```python
from build123d import *

# Parameters (mm, degrees)
F0_R      = 15.875
F0_R_2    = 12.7
F1_DEPTH  = 6.35
F2_W      = 31.75
F2_H      = 25.4
F3_DEPTH  = 6.35
F4_W      = 31.75
F4_H      = 6.35
F5_DEPTH  = 12.7
F6_W      = 19.05
F6_H      = 3.175
F7_DEPTH  = 6.35
F8_R      = 1.27
F9_R      = 12.7
F10_DEPTH = 6.35
F12_DEPTH = 6.35
F13_R     = 3.175
F14_DEPTH = 6.35


with BuildPart() as f1:
    # F0 (on Top) → F1 (new body)
    with BuildSketch(Plane.XY):
        Circle(F0_R)
        Circle(F0_R_2, mode=Mode.SUBTRACT)
    extrude(amount=F1_DEPTH)

    # F2 (on Top) → F3 (join)
    with BuildSketch(Plane.XY):
        with Locations((0, 12.7)):
            Rectangle(F2_W, F2_H)
    extrude(amount=F3_DEPTH)

    # F4 (on face) → F5 (join)
    with BuildSketch(Plane.XY.offset(6.35)):
        with Locations((0, 22.225)):
            Rectangle(F4_W, F4_H)
    extrude(amount=F5_DEPTH)

    # F6 (on face) → F7 (cut, through all)
    with BuildSketch(Plane(origin=(0, 25.4, 0), x_dir=(-1, 0, 0), z_dir=(0, 1, 0))):
        with Locations((0, 12.3825)):
            Rectangle(F6_W, F6_H)
    extrude(amount=-F7_DEPTH, mode=Mode.SUBTRACT)

    # F8
    f8_edges = [f1.edges().sort_by_distance(p)[0] for p in [
        (-9.525, 22.225, 13.97),
        (9.525, 22.225, 13.97),
        (9.525, 22.225, 10.795),
        (-9.525, 22.225, 10.795),
        (15.875, 22.225, 19.05),
        (-15.875, 22.225, 19.05),
    ]]
    fillet(f8_edges, radius=F8_R)

    # F9 (on face) → F10 (join)
    with BuildSketch(Plane(origin=(0, 0, 0), x_dir=(1, 0, 0), z_dir=(0, 0, -1))):
        Circle(F9_R)
    extrude(amount=-F10_DEPTH)

    # F11 (on face) → F12 (join)
    with BuildSketch(Plane(origin=(0, 0, 0), x_dir=(1, 0, 0), z_dir=(0, 0, -1))):
        with BuildLine():
            ThreePointArc((-15.370375, 3.970791), (-9.720579, 12.550935), (0, 15.875))
            ThreePointArc((0, 15.875), (-7.45355, 19.469551), (-9.281448, 27.540177))
            Line((-9.281448, 27.540177), (-15.370375, 3.970791))
        make_face()
        with BuildLine():
            ThreePointArc((0, 15.875), (6.735192, 18.664808), (9.525, 25.4))
            ThreePointArc((9.525, 25.4), (9.463916, 26.476995), (9.281448, 27.540177))
            ThreePointArc((9.281448, 27.540177), (0, 34.925), (-9.281448, 27.540177))
            ThreePointArc((-9.281448, 27.540177), (-7.45355, 19.469551), (0, 15.875))
        make_face()
        with BuildLine():
            ThreePointArc((9.281448, 27.540177), (9.463916, 26.476995), (9.525, 25.4))
            ThreePointArc((9.525, 25.4), (6.735192, 18.664808), (0, 15.875))
            ThreePointArc((0, 15.875), (9.720579, 12.550935), (15.370375, 3.970791))
            Line((15.370375, 3.970791), (9.281448, 27.540177))
        make_face()
    extrude(amount=-F12_DEPTH)

    # F13 (on face) → F14 (cut, through all)
    with BuildSketch(Plane.XY.offset(6.35)):
        with Locations((0, -25.4)):
            Circle(F13_R)
    extrude(amount=-F14_DEPTH, mode=Mode.SUBTRACT)


solid = f1.part
```
Read the model definition and answer for the solid it produces. Units are mm, in the model's axes. A direction names the side the tool comes from. Round coordinates to 2 decimals unless told otherwise and drop trailing zeros. Write each loop counter-clockwise with the first axis right and the second up, starting at its lowest first coordinate (ties: lowest second). Pieces come first, ordered by that corner, then holes. Notation, with made-up numbers: M 13,0.5 L 55,0.5 A23 ccw 55,8.5 Z; hole C -40,5 d1. An arc over 180 degrees is marked long. One line per item, written item: value.
Q1. Find section A-A on x = 0. Write down the section's boundary in (y, z) (3 decimals).
Data:
outline: M -34.925,0 L -28.575,0 L -28.575,6.35 L -34.925,6.35 Z; M -22.225,0 L 25.4,0 L 25.4,10.795 L 19.05,10.795 L 19.05,6.35 L -22.225,6.35 Z; M 19.05,13.97 L 25.4,13.97 L 25.4,19.05 L 19.05,19.05 Z
Q2. For a pull along Z with two mould halves and no side action, classify faces 4 (the cylindrical face through (15.49, 22.27, 18.69)), 5 (the flat face through (15.875, 15, 5)), 6 (the cylindrical face through (-9.16, 22.18, 13.59)) as +Z half, -Z half, draft (parallel to the pull), parting line (faces both ways), or undercut.
Data:
face 4: +Z half
face 5: draft
face 6: undercut
Q3. Find section C-C on z = 3.25. Write down the section's boundary in (x, y) (3 decimals), plus the area to 3 significant figures.
Data:
outline: M -15.875,0 A15.875 ccw -15.37,-3.971 L -9.281,-27.54 A9.525 ccw 9.281,-27.54 L 15.37,-3.971 A15.875 ccw 15.875,0 L 15.875,25.4 L -15.875,25.4 Z; hole C 0,-25.4 d6.35
area: 1,580 mm2
Q4. Find section D-D on y = -25.4. Write down the section's boundary in (x, z) (3 decimals).
Data:
outline: M -9.834,0 L -3.175,0 L -3.175,6.35 L -9.834,6.35 Z; M 3.175,0 L 9.834,0 L 9.834,6.35 L 3.175,6.35 Z
Q5. Flat-ended cylindrical pins translate along their axes: pin 1 Ø16 at (x, y) = (0, -4) entering from +Z; pin 2 Ø4 at (x, y) = (0, -25.4) entering from +Z; pin 3 Ø1 at (y, z) = (-28, 3.5) entering from +X. Find the tip coordinate at first contact, or state that the pin passes through.
Data:
pin 1: z = 6.35
pin 2: through
pin 3: x = 9.29
Q6. Straight lines are drawn through the part: line 1 (Y direction, x = 14, z = 6.5); line 2 (Z direction, x = -4.5, y = -30); line 3 (X direction, y = -7, z = 2.5). For each, find the intervals that lie inside material, in ascending order. Write a range as [from, to].
Data:
line 1: [19.05, 25.4]
line 2: [0, 6.35]
line 3: [-14.59, 14.59]
Q7. Find section B-B on y = 21. Write down the section's boundary in (x, z) (3 decimals).
Data:
outline: M -15.875,0 L 15.875,0 L 15.875,17.78 A1.27 ccw 14.605,19.05 L -14.605,19.05 A1.27 ccw -15.875,17.78 Z; hole M -9.525,12.065 A1.27 ccw -8.255,10.795 L 8.255,10.795 A1.27 ccw 9.525,12.065 L 9.525,12.7 A1.27 ccw 8.255,13.97 L -8.255,13.97 A1.27 ccw -9.525,12.7 Z
Q8. Which of the six approach directions +Z, -Z, +X, -X, +Y, -Y give full straight-line access (tool end or side, diameter ignored) to faces 1 (the flat face through (0, 22, 13.97)), 2 (the cylindrical face through (15.745, -2.029, 3.131)), 3 (the flat face through (0, 19.05, 15))?
Data:
face 1: +Y, -Y
face 2: +Z, -Z, +X, -Y
face 3: +Z, +X, -X, -Y
